from build123d import *

# Parameters (mm, degrees)
F0_W     = 40
F0_H     = 48
F0_R     = 4.5
F0_R_2   = 2
F0_W_2   = 11.5
F0_H_2   = 20
F1_DEPTH = 2
F2_W     = 31
F2_H     = 12
F3_DEPTH = 6
F4_W     = 1
F4_H     = 12
F5_DEPTH = 3
F6_DEPTH = 1
F7_R     = 4.99999
F8_R     = 5


# Not quite as in the source:
# - a fillet or chamfer is up to 0.001 mm smaller than in the source, because OpenCascade refuses the exact size


with BuildPart() as f1:
    # F0 (on Top) → F1 (new body)
    with BuildSketch(Plane.XY):
        with Locations((20, 24)):
            Rectangle(F0_W, F0_H)
        with Locations((10.25, 13.5)):
            Circle(F0_R, mode=Mode.SUBTRACT)
        with Locations((10.25, 22.5)):
            Circle(F0_R_2, mode=Mode.SUBTRACT)
        with Locations((35.5, 6)):
            Circle(F0_R_2, mode=Mode.SUBTRACT)
        with Locations((28.75, 22.5)):
            Rectangle(F0_W_2, F0_H_2, mode=Mode.SUBTRACT)
        with Locations((10.25, 31.5)):
            Circle(F0_R, mode=Mode.SUBTRACT)
        with Locations((34, 39)):
            Circle(F0_R_2, mode=Mode.SUBTRACT)
    extrude(amount=F1_DEPTH)

    # F2 (on face) → F3 (join)
    with BuildSketch(Plane(origin=(0, 48, 0), x_dir=(-1, 0, 0), z_dir=(0, 1, 0))):
        with Locations((-25.5, -4)):
            Rectangle(F2_W, F2_H)
    extrude(amount=F3_DEPTH)

    # F4 (on face) → F5 (cut)
    with BuildSketch(Plane(origin=(0, 54, 0), x_dir=(-1, 0, 0), z_dir=(0, 1, 0))):
        with Locations((-20, -4)):
            Rectangle(F4_W, F4_H)
        with Locations((-31, -4)):
            Rectangle(F4_W, F4_H)
    extrude(amount=-F5_DEPTH, mode=Mode.SUBTRACT)

    # F6 (add): a face of the model
    f6_faces = [f1.faces().sort_by_distance(p)[0] for p in [
        (40, 24, 1),
    ]]
    extrude(f6_faces, amount=F6_DEPTH)

    # F7 (radius 5 in the source; OpenCascade refuses exactly that, so slightly less here)
    f7_edges = [f1.edges().sort_by_distance(p)[0] for p in [
        (10, 48, 1),
        (0, 48, 1),
    ]]
    fillet(f7_edges, radius=F7_R)

    # F8
    f8_edges = [f1.edges().sort_by_distance(p)[0] for p in [
        (41, 54, -4),
    ]]
    fillet(f8_edges, radius=F8_R)


solid = f1.part
Build history of the part. All positions in model axes, mm. A direction names the side the tool comes from. Give positions to 0.01 mm unless a question says otherwise; leave off trailing zeros. Loops run counter-clockwise (first coordinate to the right, second up) from the corner with the lowest first, then second, coordinate; pieces in that order, holes last. Notation, with made-up numbers: (18.25, 23.5) - (71.25, 23.5) arc R36 ccw to (71.25, 62.5) - close; hole circle Ø2 at (-7.75, -17.75). An arc over 180 degrees is marked (long way). Write item = value, one per line. Start each with the question number.
1) Pull direction Y, two halves, no side cores. Call faces 1 (the flat face through (19.5, 53, -4)), 2 (the flat face through (26, 48, -5)), 3 (the flat face through (34.5, 22, 1)), 4 (the cylindrical face through (8.663, 21.283, 0.986)): +Y half, -Y half, draft (parallel to the pull), parting line (faces both ways), or undercut.
2) Band-saw the part on C-C on y = 11. Give the cut face in (x, z).
3) Drop flat-ended pins along their axis: pin 1 Ø11.5 at (x, y) = (10.25, 31.5) entering from -Z; pin 2 Ø1.5 at (y, z) = (52, -2.5) entering from -X; pin 3 Ø0.9 at (y, z) = (53, -2.5) entering from +X. Give the stop position or say it passes through.
4) Band-saw the part on A-A on y = 31.5. Give the cut face in (x, z), plus the area to 3 significant figures.
5) Band-saw the part on B-B on z = -4.75. Give the cut face in (x, y).
6) Tool access for faces 5 (the flat face through (20.5, 53, -4)), 6 (the cylindrical face through (2, 47, 1)), 7 (the flat face through (29, 32.5, 1)): list every direction of +Z, -Z, +X, -X, +Y, -Y with a clear straight run to the whole face (end or side of a thin tool).
7) Band-saw the part on D-D on x = 11. Give the cut face in (y, z), plus the area to 3 significant figures.
8) Probe probe 1 along Y at (x, z) = (10.25, 0.7); probe 2 along Y at (x, z) = (35.5, 0.4); probe 3 along Z at (x, y) = (28.5, 36.5). List the from-to ranges inside material, lowest first. Write a range as from..to.
Final values:
q1.face_1 = draft
q1.face_2 = -Y half
q1.face_3 = undercut
q1.face_4 = undercut
q2.outline = (0, 0) - (6.51, 0) - (6.51, 2) - (0, 2) - close; (13.99, 0) - (41, 0) - (41, 2) - (13.99, 2) - close
q3.pin_1 = 0
q3.pin_2 = 10
q3.pin_3 = 39.52
q4.outline = (0, 0) - (5.75, 0) - (5.75, 2) - (0, 2) - close; (14.75, 0) - (23, 0) - (23, 2) - (14.75, 2) - close; (34.5, 0) - (41, 0) - (41, 2) - (34.5, 2) - close
q4.area = 41.0 mm²
q5.outline = (10, 48) - (41, 48) - (41, 49) arc R5 ccw to (36, 54) - (31.5, 54) - (31.5, 51) - (30.5, 51) - (30.5, 54) - (20.5, 54) - (20.5, 51) - (19.5, 51) - (19.5, 54) - (10, 54) - close
q6.face_5 = +Z, -Z, +Y
q6.face_6 = +Z, -Z, -X, +Y
q6.face_7 = +Z, -Z
q7.outline = (0, 0) - (9.06, 0) - (9.06, 2) - (0, 2) - close; (17.94, 0) - (20.65, 0) - (20.65, 2) - (17.94, 2) - close; (24.35, 0) - (27.06, 0) - (27.06, 2) - (24.35, 2) - close; (35.94, 0) - (48, 0) - (48, -10) - (54, -10) - (54, 2) - (35.94, 2) - close
q7.area = 125 mm²
q8.probe_1 = 0..9, 18..20.5, 24.5..27, 36..54
q8.probe_2 = 0..4, 8..37.68, 40.32..54
q8.probe_3 = 0..2
